Part model, mm, in its own coordinate system. Coordinates: 2 decimals unless noted, no trailing zeros. One line per question, with ' | ' between items. Start each with the question number.
1) Drop flat-ended pins along their axis: pin 1 (8 mm diameter, centred on x = 481, z = 0, fed in from +Y); pin 2 (2 mm diameter, centred on y = -9.5, z = -6.5, fed in from -X). Give the stop position or say it passes through.
2) Probe L1, parallel to Y at x = 214, z = -9; L2, parallel to Y at x = 10, z = -13.25; L3, parallel to Z at x = 347, y = 13.7. List the from-to ranges inside material, lowest first. Write a range as from..to.
3) Cut at A-A (x = 362.5). Count the separate pieces of the cut face and the enclosed holes in it, plus the area to 3 significant figures.
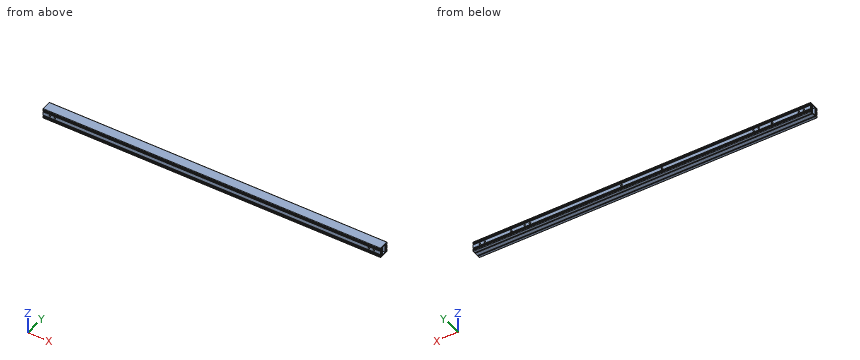
from build123d import *

# Parameters (mm, degrees)
SKETCH_1_W             = 23.5
SKETCH_1_H             = 12
EXTRUDE_1_DEPTH        = 501
HOLE_WIZARD_M6_1_D     = 5
HOLE_WIZARD_M6_1_DEPTH = 15
HOLE_WIZARD_M6_1_TIP   = 1.502151548
HOLE_WIZARD_M6_2_D     = 5
HOLE_WIZARD_M6_2_DEPTH = 15
HOLE_WIZARD_M6_2_TIP   = 1.502151548
HOLE_WIZARD_M6_3_D     = 5
HOLE_WIZARD_M6_3_DEPTH = 15
HOLE_WIZARD_M6_3_TIP   = 1.502151548


with BuildPart() as part:
    # Sketch 1 → Extrude 1 (new, symmetric)
    with BuildSketch(Plane(origin=(0, 0, 0), x_dir=(0, 0, -1), z_dir=(1, 0, 0))):
        with BuildLine():
            Line((-14, 15), (-11.5, 15))
            Line((-11.5, 15), (-11.5, 13.5))
            Line((-11.5, 13.5), (-11.4, 13.5))
            ThreePointArc((-11.4, 13.5), (-11.117157288, 13.382842712), (-11, 13.1))
            Line((-11, 13.1), (-11, 12))
            Line((-11, 12), (-9.5, 12))
            Line((-9.5, 12), (-9.5, 15))
            Line((-9.5, 15), (-8, 15))
            Line((-8, 15), (-8, 12.5))
            Line((-8, 12.5), (-5, 12.5))
            Line((-5, 12.5), (-5, 15))
            Line((-5, 15), (5, 15))
            Line((5, 15), (5, 12.5))
            Line((5, 12.5), (8, 12.5))
            Line((8, 12.5), (8, 15))
            Line((8, 15), (9.5, 15))
            Line((9.5, 15), (9.5, 12))
            Line((9.5, 12), (11, 12))
            Line((11, 12), (11, 13.1))
            ThreePointArc((11, 13.1), (11.117157288, 13.382842712), (11.4, 13.5))
            Line((11.4, 13.5), (11.5, 13.5))
            Line((11.5, 13.5), (11.5, 15))
            Line((11.5, 15), (14, 15))
            ThreePointArc((14, 15), (14.707106781, 14.707106781), (15, 14))
            Line((15, 14), (15, 8))
            Line((15, 8), (12.5, 8))
            Line((12.5, 8), (12.5, 5))
            Line((12.5, 5), (15, 5))
            Line((15, 5), (15, -5))
            Line((15, -5), (12.5, -5))
            Line((12.5, -5), (12.5, -8))
            Line((12.5, -8), (15, -8))
            Line((15, -8), (15, -14))
            ThreePointArc((15, -14), (14.707106781, -14.707106781), (14, -15))
            Line((14, -15), (11.5, -15))
            Line((11.5, -15), (11.5, -13.5))
            Line((11.5, -13.5), (11.4, -13.5))
            ThreePointArc((11.4, -13.5), (11.117157288, -13.382842712), (11, -13.1))
            Line((11, -13.1), (11, -12))
            Line((11, -12), (9.5, -12))
            Line((9.5, -12), (9.5, -15))
            Line((9.5, -15), (8, -15))
            Line((8, -15), (8, -12.5))
            Line((8, -12.5), (5, -12.5))
            Line((5, -12.5), (5, -15))
            Line((5, -15), (-5, -15))
            Line((-5, -15), (-5, -12.5))
            Line((-5, -12.5), (-8, -12.5))
            Line((-8, -12.5), (-8, -15))
            Line((-8, -15), (-9.5, -15))
            Line((-9.5, -15), (-9.5, -12))
            Line((-9.5, -12), (-11, -12))
            Line((-11, -12), (-11, -13.1))
            ThreePointArc((-11, -13.1), (-11.117157288, -13.382842712), (-11.4, -13.5))
            Line((-11.4, -13.5), (-11.5, -13.5))
            Line((-11.5, -13.5), (-11.5, -15))
            Line((-11.5, -15), (-14, -15))
            ThreePointArc((-14, -15), (-14.707106781, -14.707106781), (-15, -14))
            Line((-15, -14), (-15, 14))
            ThreePointArc((-15, 14), (-14.707106781, 14.707106781), (-14, 15))
        make_face()
        with BuildLine():
            Line((12, -10.5), (12, -8.5))
            ThreePointArc((12, -8.5), (11.853553391, -8.146446609), (11.5, -8))
            Line((11.5, -8), (-11.5, -8))
            ThreePointArc((-11.5, -8), (-11.853553391, -8.146446609), (-12, -8.5))
            Line((-12, -8.5), (-12, -10.5))
            ThreePointArc((-12, -10.5), (-11.853553391, -10.853553391), (-11.5, -11))
            Line((-11.5, -11), (11.5, -11))
            ThreePointArc((11.5, -11), (11.853553391, -10.853553391), (12, -10.5))
        make_face(mode=Mode.SUBTRACT)
        with BuildLine():
            Line((-11.5, 11), (11.5, 11))
            ThreePointArc((11.5, 11), (11.853553391, 10.853553391), (12, 10.5))
            Line((12, 10.5), (12, 8.5))
            ThreePointArc((12, 8.5), (11.853553391, 8.146446609), (11.5, 8))
            Line((11.5, 8), (-11.5, 8))
            ThreePointArc((-11.5, 8), (-11.853553391, 8.146446609), (-12, 8.5))
            Line((-12, 8.5), (-12, 10.5))
            ThreePointArc((-12, 10.5), (-11.853553391, 10.853553391), (-11.5, 11))
        make_face(mode=Mode.SUBTRACT)
        Rectangle(SKETCH_1_W, SKETCH_1_H, mode=Mode.SUBTRACT)
    extrude(amount=EXTRUDE_1_DEPTH, both=True)

    # Hole Wizard M6 _1
    with Locations(Plane.XZ.offset(15)):
        with Locations((-481, 0), (-466, 0), (466, 0), (481, 0)):
            Hole(HOLE_WIZARD_M6_1_D / 2, depth=HOLE_WIZARD_M6_1_DEPTH)
            with Locations((0, 0, -(HOLE_WIZARD_M6_1_DEPTH + HOLE_WIZARD_M6_1_TIP / 2))):  # 118° drill point
                Cone(0, HOLE_WIZARD_M6_1_D / 2, HOLE_WIZARD_M6_1_TIP, mode=Mode.SUBTRACT)

    # Hole Wizard M6 _2
    with Locations(Plane(origin=(0, 15, 0), x_dir=(-1, 0, 0), z_dir=(0, 1, 0))):
        with Locations((-481, 0), (-466, 0), (466, 0), (481, 0)):
            Hole(HOLE_WIZARD_M6_2_D / 2, depth=HOLE_WIZARD_M6_2_DEPTH)
            with Locations((0, 0, -(HOLE_WIZARD_M6_2_DEPTH + HOLE_WIZARD_M6_2_TIP / 2))):  # 118° drill point
                Cone(0, HOLE_WIZARD_M6_2_D / 2, HOLE_WIZARD_M6_2_TIP, mode=Mode.SUBTRACT)

    # Hole Wizard M6 _3
    with Locations(Plane(origin=(0, 15, 0), x_dir=(-1, 0, 0), z_dir=(0, 1, 0))):
        with Locations((387, 0), (347, 0), (60, 0), (-60, 0), (-347, 0), (-387, 0), (332, 0), (-332, 0)):
            Hole(HOLE_WIZARD_M6_3_D / 2, depth=HOLE_WIZARD_M6_3_DEPTH)
            with Locations((0, 0, -(HOLE_WIZARD_M6_3_DEPTH + HOLE_WIZARD_M6_3_TIP / 2))):  # 118° drill point
                Cone(0, HOLE_WIZARD_M6_3_D / 2, HOLE_WIZARD_M6_3_TIP, mode=Mode.SUBTRACT)


solid = part.part
Reported:
1) pin 1: stops at y = 15 | pin 2: passes through
2) L1: y = -15..-11, -8..-6, 6..8, 11..15 | L2: y = -15..-8, -5..5, 8..15 | L3: z = -15..-11.5, -9.5..-8, -5..-2.5, 2.5..5, 8..9.5, 11.5..15
3) separate pieces: 1 | enclosed holes: 3 | area: 407 mm²
